```python
from build123d import *

# Parameters (mm, degrees)
BOSS_EXTRUDE1_DEPTH = 10
SKETCH2_R           = 1.5
BOSS_EXTRUDE2_DEPTH = 5


with BuildPart() as part:
    # Sketch1 → Boss-Extrude1 (new body)
    with BuildSketch(Plane.XY):
        Polygon((0, 0), (0, -6.709191333), (-4.597281239, -11.306472572), (-57.229872555, -11.306472572), (-83.792838338, -11.306472572), (-90.706486966, -11.306472572), (-90.706486966, -4.193244583), (-63.77964494, -1.677297833), (-49.58847144, -1.677297833), (-35.945470397, -1.677297833), (-30.913576897, -6.709191333), (-12.549158145, -6.709191333), (-9.194562479, -3.354595666), (-9.194562479, 0), (-4.597281239, 4.597281239), align=None)
    extrude(amount=BOSS_EXTRUDE1_DEPTH)

    # Sketch2 → Boss-Extrude2 (add)
    with BuildSketch(Plane(origin=(0, 0, 0), x_dir=(-1, 0, 0), z_dir=(0, 0, -1))):
        with Locations(Location((3.981479871, -1.591444595, 0), (0, 0, 180))):
            Circle(SKETCH2_R)
    extrude(amount=BOSS_EXTRUDE2_DEPTH)


solid = part.part
```
The model under review builds one solid part; all positions refer to its coordinate system, in mm. A direction names the side the tool comes from. Round coordinates to 2 decimals unless told otherwise and drop trailing zeros. Loops run counter-clockwise (first coordinate to the right, second up) from the corner with the lowest first, then second, coordinate; pieces in that order, holes last. Notation, with made-up numbers: (60, 47) - (92, 47) arc R21 cw to (92, 71) - close; hole circle Ø7 at (28.25, -31.5). An arc over 180 degrees is marked (long way). Use a Markdown table: item, result. Add a question column.
Q1. Add section B-B (z = 4). State the section outline as (x, y) points, plus the area to 3 significant figures.
Q2. Insertion check: pin 1 Ø3 at (y, z) = (0.5, -1) entering from -X; pin 2 Ø1.5 at (x, z) = (-78, -1.5) entering from -Y; pin 3 Ø1 at (x, y) = (-34.5, -2.5) entering from -Z; pin 4 Ø5 at (x, z) = (-22.5, 2.5) entering from +Y. Each pin has a flat end and moves straight along its axis. Give the tip position at first contact, or say it passes through.
Q3. Add section C-C (x = -23). State the section outline as (y, z) points.
Q4. For probe 1 along X at (y, z) = (-1.5, -0.5); probe 2 along Z at (x, y) = (-36, -10); probe 3 along Y at (x, z) = (-14.5, 5.5), list the stretches that pass through material, from the lowest coordinate up.
Q5. Machinability: for faces 1 (the face through (-50, -1.677, 5)), 2 (the face through (-22, -6.709, 5)), 3 (the face through (-4.18, -3.08, -2.46)), which of the approach directions +Z, -Z, +X, -X, +Y, -Y give a long, thin tool a straight path to every point of the face, cutting with its end or side? Answer none if there is none.
Q6. Add section D-D (y = 1.25). State the section outline as (x, z) points.
Q7. Add section A-A (y = -5.25). State the section outline as (x, z) points, plus the area to 3 significant figures.
Q8. The part is to be moulded in two halves that separate along X. For faces 4 (the face through (-10.9, -5.06, 4.93)), 5 (the face through (-2.27, -8.98, 4.93)), 6 (the face through (-45, -7, 10)), say which applies: pulls with the +X half, pulls with the -X half, needs draft (parallel to the pull), parting line crosses it, or undercut.
Worked answers:
| question | item | result |
|---|---|---|
| 1 | outline | (-90.71, -11.31) - (-4.6, -11.31) - (0, -6.71) - (0, 0) - (-4.6, 4.6) - (-9.19, 0) - (-9.19, -3.35) - (-12.55, -6.71) - (-30.91, -6.71) - (-35.95, -1.68) - (-63.78, -1.68) - (-90.71, -4.19) - close |
| 1 | area | 749 mm² |
| 2 | pin 1 | x = -9.19 |
| 2 | pin 2 | through |
| 2 | pin 3 | z = 0 |
| 2 | pin 4 | y = -6.71 |
| 3 | outline | (-11.31, 0) - (-6.71, 0) - (-6.71, 10) - (-11.31, 10) - close |
| 4 | probe 1 | -5.48 to -2.48 |
| 4 | probe 2 | 0 to 10 |
| 4 | probe 3 | -11.31 to -6.71 |
| 5 | face 1 | +Z, -Z, -X, +Y |
| 5 | face 2 | +Z, -Z, +Y |
| 5 | face 3 | -Z |
| 6 | outline | (-7.94, 0) - (-1.25, 0) - (-1.25, 10) - (-7.94, 10) - close |
| 7 | outline | (-90.71, 0) - (-32.37, 0) - (-32.37, 10) - (-90.71, 10) - close; (-11.09, 0) - (0, 0) - (0, 10) - (-11.09, 10) - close |
| 7 | area | 694 mm² |
| 8 | face 4 | undercut |
| 8 | face 5 | pulls with the +X half |
| 8 | face 6 | needs draft |
